```python
from build123d import *

# Parameters (mm, degrees)
F0_W     = 20
F0_H     = 231
F1_DEPTH = 8.75
F2_SIZE2 = 17.49999
F2_SIZE  = 17.49999
F3_SIZE2 = 33.49999
F3_SIZE  = 17.49999
F4_SIZE2 = 17.49999
F4_SIZE  = 19.99999


# Not quite as in the source:
# - a fillet or chamfer is up to 0.001 mm smaller than in the source, because OpenCascade refuses the exact size


with BuildPart() as f1:
    # F0 (on Top) → F1 (new body, symmetric)
    with BuildSketch(Plane.XY):
        Rectangle(F0_W, F0_H)
    extrude(amount=F1_DEPTH, both=True)

    # F2 (size 17.5 and 17.5 in the source; OpenCascade refuses exactly that, so slightly less here)
    f2_edges = [f1.edges().sort_by_distance(p)[0] for p in [
        (0, -115.5, 8.75),
    ]]
    chamfer(f2_edges, length=F2_SIZE, length2=F2_SIZE2)

    # F3 (size 17.5 and 33.5 in the source; OpenCascade refuses exactly that, so slightly less here)
    f3_edges = [f1.edges().sort_by_distance(p)[0] for p in [
        (0, 115.5, 8.75),
    ]]
    f3_side = f1.faces().sort_by_distance((0, 115.5, 0))[0]
    chamfer(f3_edges, length=F3_SIZE, length2=F3_SIZE2, reference=f3_side)

    # F4 (size 20 and 17.5 in the source; OpenCascade refuses exactly that, so slightly less here)
    f4_edges = [f1.edges().sort_by_distance(p)[0] for p in [
        (-10, -8, 8.75),
    ]]
    f4_side = f1.faces().sort_by_distance((0, -8, 8.75))[0]
    chamfer(f4_edges, length=F4_SIZE, length2=F4_SIZE2, reference=f4_side)


solid = f1.part
```
For this review, take the finished solid that the model builds, in its own axes (mm). Round coordinates to 2 decimals unless told otherwise and drop trailing zeros. Loops run counter-clockwise (first coordinate to the right, second up) from the corner with the lowest first, then second, coordinate; pieces in that order, holes last.
(1) We need section C-C (z = -1.5). Give the boundary of the cut face in (x, y).
Returned:
outline: (-1.71, -108.25) - (10, -108.25) - (10, 101.62) - (-1.71, 101.62) - close
(2) Clearance check with flat-ended pins moving along their axes: P1, Ø5, axis at x = -2, y = 69, coming from the +Z side; P2, Ø6, axis at x = 7.5, z = 7, coming from the +Y side; P3, Ø1.5, axis at x = 4, z = 3.5, coming from the -Y side. State where each tip first meets the part, or that it passes through.
Returned:
P1: stops at z = 0.44
P2: stops at y = 91.09
P3: stops at y = -104
(3) Wall thickness on line 1 along X through (y, z) = (-53, 4.5); line 2 along Z through (x, y) = (7, -72) (3 decimals); line 3 along Y through (x, z) = (7.5, 6): over which ranges is each line inside the solid? List them lowest first.
Returned:
line 1: x = 5.14 to 10
line 2: z = -8.75 to 6.125
line 3: y = -100.75 to 87.26
